Read the model definition and answer for the solid it produces. Units are mm, in the model's axes. Coordinates: 2 decimals unless noted, no trailing zeros. Loops run counter-clockwise (first coordinate to the right, second up) from the corner with the lowest first, then second, coordinate; pieces in that order, holes last. Notation, with made-up numbers: (67.5, 74.5) -> (118.5, 74.5) arc R15 ccw to (118.5, 92.5) -> close; hole circle Ø9 at (-32, 74). An arc over 180 degrees is marked (long way). One line per question, with ' | ' between items. Start each with the question number.
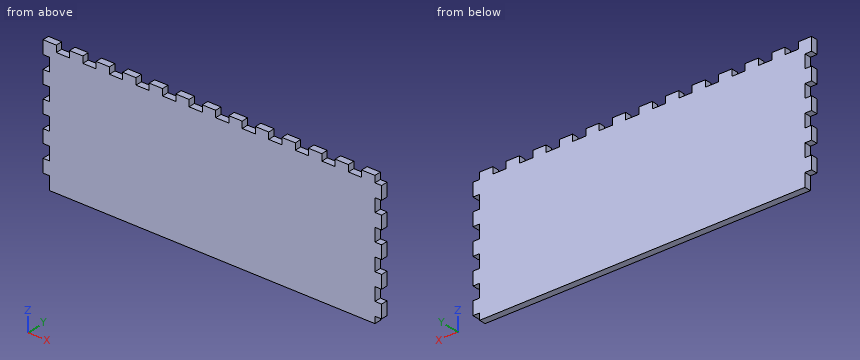
```python
from build123d import *

# Parameters (mm, degrees)
SKETCH051_W             = 95
SKETCH051_H             = 250
PAD035_DEPTH            = 5
SKETCH056_W             = 10
SKETCH056_H             = 5
PAD040_DEPTH            = 5
LINEARPATTERN031_COUNT  = 5
LINEARPATTERN031_PITCH  = 20
SKETCH062_W             = 10
SKETCH062_H             = 5
PAD043_DEPTH            = 5
LINEARPATTERN037_COUNT  = 13
LINEARPATTERN037_PITCH  = 20
SKETCH069_W             = 10
SKETCH069_H             = 5
POCKET022_DEPTH         = 5
LINEARPATTERN044_COUNT  = 5
LINEARPATTERN044_PITCH  = 20
BODY014_PITCH_ANGLE     = -90
BODY014_PLACEMENT_ANGLE = 90


with BuildPart() as part:
    # Sketch051 → Pad035 (new body)
    with BuildSketch(Plane.XY):
        Rectangle(SKETCH051_W, SKETCH051_H)
    extrude(amount=PAD035_DEPTH)

    # Sketch056 (on DatumPlane) → Pad040 (join)
    with BuildSketch(Plane.XZ.offset(125)):
        with Locations((-37.5, 2.5)):
            Rectangle(SKETCH056_W, SKETCH056_H)
    pad040 = extrude(amount=PAD040_DEPTH)

    # LinearPattern031: Pad040 ×5
    with Locations(*[(i * LINEARPATTERN031_PITCH, 0, 0) for i in range(1, LINEARPATTERN031_COUNT)]):
        add(pad040)

    # Sketch062 (on DatumPlane) → Pad043 (join)
    with BuildSketch(Plane.YZ.offset(47.5)):
        with Locations((-120, 2.5)):
            Rectangle(SKETCH062_W, SKETCH062_H)
    pad043 = extrude(amount=PAD043_DEPTH)

    # LinearPattern037: Pad043 ×13
    with Locations(*[(0, i * LINEARPATTERN037_PITCH, 0) for i in range(1, LINEARPATTERN037_COUNT)]):
        add(pad043)

    # Sketch069 (on DatumPlane) → Pocket022 (cut)
    with BuildSketch(Plane(origin=(0, 125, 0), x_dir=(-1, 0, 0), z_dir=(0, 1, 0))):
        with Locations((-37.5, 2.5)):
            Rectangle(SKETCH069_W, SKETCH069_H)
    pocket022 = extrude(amount=-POCKET022_DEPTH, mode=Mode.SUBTRACT)

    # LinearPattern044: Pocket022 ×5
    with Locations(*[(-i * LINEARPATTERN044_PITCH, 0, 0) for i in range(1, LINEARPATTERN044_COUNT)]):
        add(pocket022, mode=Mode.SUBTRACT)


with BuildPart() as part_1:
    # Body014 pitch: moved
    add(part.part.rotate(Axis((0, 0, 0), (0, 1, 0)), BODY014_PITCH_ANGLE))


with BuildPart() as part_2:
    # Body014 placement: moved
    add(part_1.part.moved(Location((125, 150, 152.5))).rotate(Axis((125, 150, 152.5), (0, 0, 1)), BODY014_PLACEMENT_ANGLE))


solid = part_2.part
```
(1) Find the intervals of material crossed by probe 1 along X at (y, z) = (147.3, 149); probe 2 along Z at (x, y) = (33, 148); probe 3 along X at (y, z) = (149.6, 172), in increasing order. Write a range as from..to.
(2) Each of these flat-tipped pins is pushed along its axis until it touches: pin 1 Ø1.5 at (x, y) = (252, 147) entering from -Z; pin 2 Ø2.5 at (y, z) = (147.5, 202) entering from +X; pin 3 Ø1 at (y, z) = (149, 167) entering from -X. Where does it stop, or does it pass through?
(3) Section A-A on x = 33 is taken. Write down the section's boundary in (y, z), plus the area to 3 significant figures.
(4) Section B-B on z = 152.5 is taken. Write down the section's boundary in (x, y).
Working result:
1) probe 1: x = 5..250 | probe 2: z = 105..200 | probe 3: x = 5..255
2) pin 1: stops at z = 110 | pin 2: stops at x = 250 | pin 3: stops at x = 5
3) outline: (145, 105) -> (150, 105) -> (150, 200) -> (145, 200) -> close | area: 475 mm2
4) outline: (5, 145) -> (255, 145) -> (255, 150) -> (5, 150) -> close
